Autodesk Inventor part; units mm, degrees
ref_plane "YZ Plane" through (0, 0, 0) normal (1, 0, 0) x (0, 1, 0)
ref_plane "XZ Plane" through (0, 0, 0) normal (0, 1, 0) x (-1, 0, 0)
ref_plane "XY Plane" through (0, 0, 0) normal (0, 0, 1) x (1, 0, 0)
sketch "Skizze1" plane through (0, 0, 0) normal (0, 1, 0) x (-1, 0, 0)
  circle A0 centre (0, 0) radius 8
  dimension "d0" = 16
extrude "Extrusion1" add sketch "Skizze1" along normal blind 12.2
fillet "Rundung1" radius 0.5 2 edges at (8, 12.2, 0) (8, 0, 0)
sketch "Skizze2" plane through (0, 12.2, 0) normal (0, 1, 0) x (1, 0, 0)
  circle A0 centre (0, 0) radius 6.2
  circle A1 centre (0, 0) radius 8
  dimension "d4" = 1.8
extrude "Extrusion2" cut sketch "Skizze2" against normal blind 0.5 contours A0
sketch "Skizze3" plane through (0, 0, 0) normal (0, -1, 0) x (1, 0, 0)
  circle A0 centre (0, 0) radius 7.5
extrude "Extrusion3" cut sketch "Skizze3" against normal blind 0.75
sketch "Skizze4" plane through (0, 0.75, 0) normal (0, -1, 0) x (1, 0, 0)
  circle A0 centre (0, -5) radius 0.5
  circle A1 centre (0, 5) radius 0.5
  point P0 (0, 0)
  dimension "d9" = 10
  dimension "d10" = 5
  dimension "d11" = 1
  dimension "d12" = 1
extrude "Extrusion4" add sketch "Skizze4" along normal blind 10
sketch "Skizze5" plane through (0, 0.75, 0) normal (0, -1, 0) x (1, 0, 0)
  circle A0 centre (0, -5) radius 0.5
  circle A1 centre (0, -5) radius 1.5
  circle A2 centre (0, 5) radius 0.5
  circle A3 centre (0, 5) radius 0.75
  circle A4 centre (0, 5) radius 0.5
  circle A5 centre (0, -5) radius 0.5
  point P0 (0, 0)
  dimension "d15" = 0
  dimension "d16" = 0
  dimension "d17" = 1
  dimension "d18" = 0.25
extrude "Extrusion5" cut sketch "Skizze5" against normal blind 0.1
equation "\"d12\" = d11"
properties part number "Ultraschallwandler16mm"
For this review, take the finished solid that the model builds, in its own axes (mm). A direction names the side the tool comes from. Coordinates: 2 decimals unless noted, no trailing zeros. Order: outer loops, then holes, each group sorted by start corner. A loop starts at its lowest first (then second) coordinate and runs counter-clockwise, first axis right, second up. Notation, with made-up numbers: (43.5, 62.5) - (86.5, 62.5) arc R16 ccw to (86.5, 87.5) - close; hole circle Ø10 at (39, 79). An arc over 180 degrees is marked (long way). Answer as a JSON object with one key per item and string values. Group by question number.
1. We need section A-A on z = 0. State the section outline as (x, y) points, then the cut area to 3 significant figures.
2. The part is to be moulded in two halves that separate along Z. For faces 4 (the flat face through (0, -9.25, 5)), 5 (the cylindrical face through (1.73, 6.02, 7.81)), 6 (the cylindrical face through (-7.493, 0.37, 0.33)), say which applies: pulls with the +Z half, pulls with the -Z half, needs draft (parallel to the pull), parting line crosses it, or undercut.
3. We need section D-D on y = 1.75. State the section outline as (x, z) points.
4. For faces 1 (the flat face through (0, -9.25, -5)), 2 (the flat face through (0, 0.75, 0)), 3 (the cylindrical face through (2.86, 11.95, 5.5)), list the 3-axis set-ups (+Z, -Z, +X, -X, +Y, -Y) from which the entire face can be reached by the end or side of a thin tool; tool diameter is ignored.
5. For probe 1 along Z at (x, y) = (0, 0.65); probe 2 along Z at (x, y) = (0, 0.8); probe 3 along Y at (x, z) = (4.5, 5.5), list the stretches that pass through material, from the lowest coordinate up.
6. We need section C-C on y = -2. State the section outline as (x, z) points, then the cut area to 3 significant figures.
7. Clearance check with flat-ended pins moving along their axes: P1, Ø6, axis at y = -4, z = 5, coming from the +X side; P2, Ø4, axis at x = -1.5, z = -2, coming from the -Y side; P3, Ø3, axis at x = -0.5, z = -4, coming from the +Y side. State where each tip first meets the part, or that it passes through.
Final values:
{
 "1": {"outline": "(-8, 0.5) arc R0.5 ccw to (-7.5, 0) - (-7.5, 0.75) - (7.5, 0.75) - (7.5, 0) arc R0.5 ccw to (8, 0.5) - (8, 11.7) arc R0.5 ccw to (7.5, 12.2) - (6.2, 12.2) - (6.2, 11.7) - (-6.2, 11.7) - (-6.2, 12.2) - (-7.5, 12.2) arc R0.5 ccw to (-8, 11.7) - close", "area": "178 mm²"},
 "2": {"face 4": "needs draft", "face 5": "parting line crosses it", "face 6": "undercut"},
 "3": {"outline": "circle Ø16 at (0, 0)"},
 "4": {"face 1": "+Z, -Z, +X, -X, -Y", "face 2": "-Y", "face 3": "+Y"},
 "5": {"probe 1": "-8 to -7.5, -5.5 to -4.5, 4.5 to 5.5, 7.5 to 8", "probe 2": "-8 to -6.5, -5.5 to -4.5, -3.5 to 4.25, 4.5 to 5.5, 5.75 to 8", "probe 3": "0.75 to 12.2"},
 "6": {"outline": "circle Ø1 at (0, -5); circle Ø1 at (0, 5)", "area": "1.57 mm²"},
 "7": {"P1": "x = 0.5", "P2": "y = 0.75", "P3": "y = 11.7"}
}
